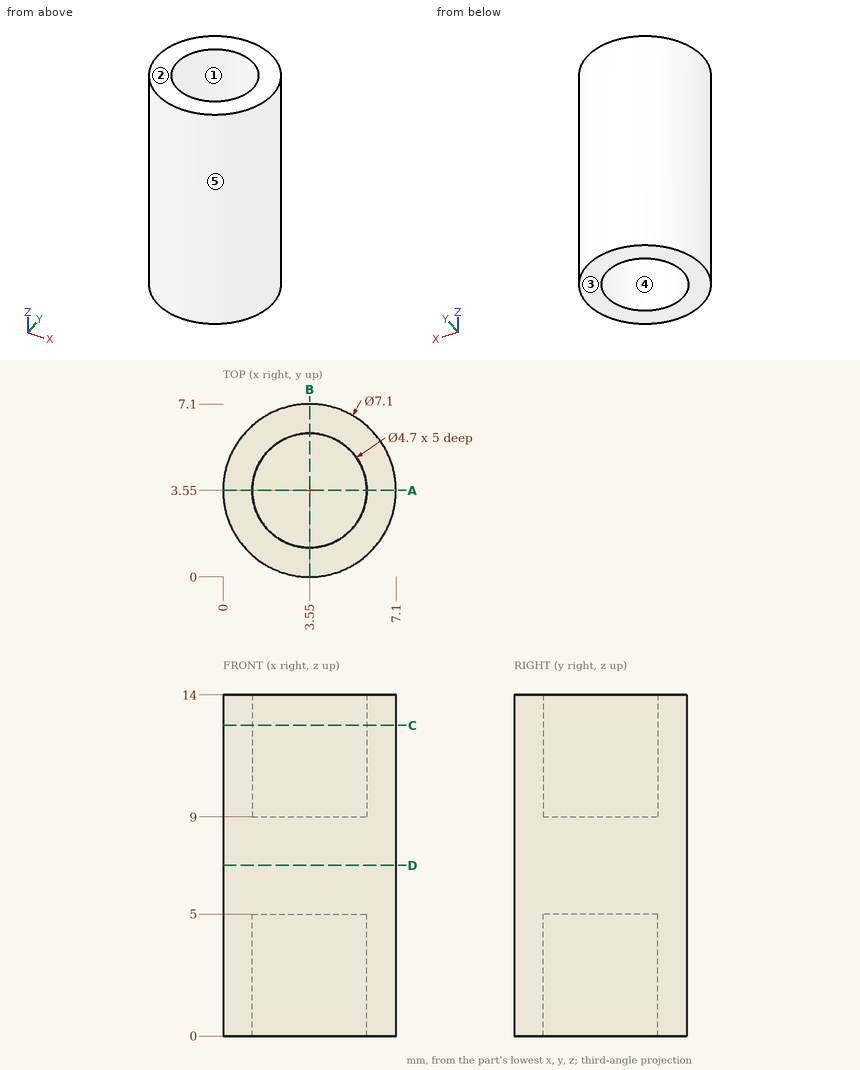
Part print with two shaded views. Sizes in mm from the minimum x, y, z corner. A direction names the side the tool comes from. Coordinates: 2 decimals unless noted, no trailing zeros. Write each loop counter-clockwise with the first axis right and the second up, starting at its lowest first coordinate (ties: lowest second). Pieces come first, ordered by that corner, then holes.
(1) Drill centre lines: line 1 (X direction, y = 3.5, z = 12.5); line 2 (Z direction, x = 2.5, y = 5); line 3 (Y direction, x = 4.5, z = 2.5). Where is each one in solid material? Low to high.
(2) Mould opens along Y. For the marked faces 3, 4 and 5 say: pulls with the +Y half, pulls with the -Y half, needs draft (parallel to the pull), parting line crosses it, or undercut.
(3) Cut at A-A on y = 3.55. List the corners of the cut face in (x, z), and give its area (3 significant figures).
(4) 3-axis set-ups, long thin cutter, end or side, ignore diameter. For the marked faces 1 and 2: which of +Z, -Z, +X, -X, +Y, -Y reach the whole face in a straight line?
(5) Pin check, flat tips, straight feed: pin 1 Ø1.5 at (x, z) = (3, 12.5) entering from +Y; pin 2 Ø1.4 at (x, y) = (3, 4) entering from -Z; pin 3 Ø3 at (x, z) = (6, 11) entering from +Y; pin 4 Ø1 at (y, z) = (5.5, 5.5) entering from +X. Stop position of each tip, or through.
(6) Cut at D-D on z = 7. List the corners of the cut face in (x, y), and give its area (3 significant figures).
(7) Cut at C-C on z = 12.75. List the corners of the cut face in (x, y).
Working result:
1. line 1: x = 0 to 1.2, 5.9 to 7.1
1. line 2: z = 5 to 9
1. line 3: y = 0.13 to 1.4, 5.7 to 6.97
2. face 3: needs draft
2. face 4: undercut
2. face 5: parting line crosses it
3. outline: (0, 0) - (1.2, 0) - (1.2, 5) - (5.9, 5) - (5.9, 0) - (7.1, 0) - (7.1, 14) - (5.9, 14) - (5.9, 9) - (1.2, 9) - (1.2, 14) - (0, 14) - close
3. area: 52.4 mm2
4. face 1: +Z
4. face 2: +Z, +X, -X, +Y, -Y
5. pin 1: stops at y = 7.1
5. pin 2: stops at z = 5
5. pin 3: stops at y = 6.97
5. pin 4: stops at x = 6.79
6. outline: circle Ø7.1 at (3.55, 3.55)
6. area: 39.6 mm2
7. outline: circle Ø7.1 at (3.55, 3.55); hole circle Ø4.7 at (3.55, 3.55)
